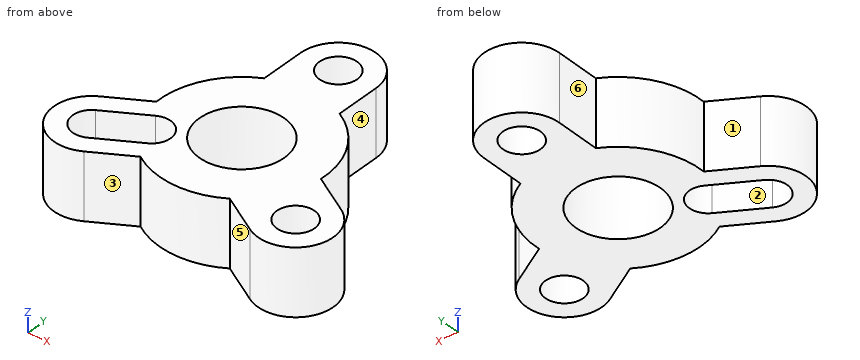
from build123d import *

# Parameters (mm, degrees)
SKETCH_1_R      = 9
SKETCH_1_R_2    = 4
EXTRUDE_1_DEPTH = 14


with BuildPart() as part:
    # Эскиз1 → Бобышка-Вытянуть1 (new body)
    with BuildSketch(Plane.XY):
        with BuildLine():
            Line((-8, 25), (-8, 15.564382416))
            ThreePointArc((-8, 15.564382416), (-15.155444566, 8.75), (-17.479150567, -0.853987978))
            Line((-17.479150567, -0.853987978), (-25.650635095, -5.57179677))
            ThreePointArc((-25.650635095, -5.57179677), (-28.578838325, -16.5), (-17.650635095, -19.42820323))
            Line((-17.650635095, -19.42820323), (-9.479150567, -14.710394438))
            ThreePointArc((-9.479150567, -14.710394438), (0, -17.5), (9.479150567, -14.710394438))
            Line((9.479150567, -14.710394438), (17.650635095, -19.42820323))
            ThreePointArc((17.650635095, -19.42820323), (28.578838325, -16.5), (25.650635095, -5.57179677))
            Line((25.650635095, -5.57179677), (17.479150567, -0.853987978))
            ThreePointArc((17.479150567, -0.853987978), (15.155444566, 8.75), (8, 15.564382416))
            Line((8, 15.564382416), (8, 25))
            ThreePointArc((8, 25), (0, 33), (-8, 25))
        make_face()
        Circle(SKETCH_1_R, mode=Mode.SUBTRACT)
        with Locations((0, 25)):
            Circle(SKETCH_1_R_2, mode=Mode.SUBTRACT)
        with Locations((21.650635095, -12.5)):
            Circle(SKETCH_1_R_2, mode=Mode.SUBTRACT)
        with BuildLine():
            Line((-14.990381057, -4.035898385), (-23.650635095, -9.035898385))
            ThreePointArc((-23.650635095, -9.035898385), (-25.11473671, -14.5), (-19.650635095, -15.964101615))
            Line((-19.650635095, -15.964101615), (-10.990381057, -10.964101615))
            ThreePointArc((-10.990381057, -10.964101615), (-9.526279442, -5.5), (-14.990381057, -4.035898385))
        make_face(mode=Mode.SUBTRACT)
    extrude(amount=EXTRUDE_1_DEPTH)


solid = part.part
Can you work these out from the model? Positions are in its coordinate system, mm. Face numbers are marked on the shaded views. A direction names the side the tool comes from. Round coordinates to 2 decimals unless told otherwise and drop trailing zeros. Write each loop counter-clockwise with the first axis right and the second up, starting at its lowest first coordinate (ties: lowest second). Pieces come first, ordered by that corner, then holes. Notation, with made-up numbers: M 26,-8 L 71,-8 A20 ccw 71,21 Z; hole C -21.5,55.25 d3. An arc over 180 degrees is marked long. Use CSV: the item, a comma, the result in double quotes.
(1) We'd pull the mould along X, two halves only. Please class the marked faces 4, 5 and 6: +X half, -X half, draft (parallel to the pull), parting line (faces both ways), or undercut.
Check values:
face 4,"+X half"
face 5,"undercut"
face 6,"-X half"
(2) Imagine slicing it at A-A (z = 1.5). Write out the boundary of the cut face in (x, y).
Check values:
outline,"M -25.65,-5.57 A8 ccw -17.65,-19.43 L -9.48,-14.71 A17.5 ccw 9.48,-14.71 L 17.65,-19.43 A8 ccw 25.65,-5.57 L 17.48,-0.85 A17.5 ccw 8,15.56 L 8,25 A8 ccw -8,25 L -8,15.56 A17.5 ccw -17.48,-0.85 Z; hole M -23.65,-9.04 A4 ccw -19.65,-15.96 L -10.99,-10.96 A4 ccw -14.99,-4.04 Z; hole C 0,0 d18; hole C 0,25 d8; hole C 21.65,-12.5 d8"
(3) I'm going to push flat-ended pins straight in: pin 1 (1 mm diameter, centred on x = -15, z = 4.5, fed in from -Y); pin 2 (4 mm diameter, centred on y = -8.5, z = 3, fed in from -X); pin 3 (2 mm diameter, centred on x = 15, z = 12.5, fed in from -Y). Where does each tip first touch, or does it pass through?
Check values:
pin 1,"y = -18.19"
pin 2,"x = -29.4"
pin 3,"y = -18.48"
(4) On a 3-axis mill with a long thin cutter (end or side, diameter ignored), from which of +Z, -Z, +X, -X, +Y, -Y can I reach the whole of each face in a straight line? I mean the marked faces 1, 2 and 3. Say none if no direction works.
Check values:
face 1,"+Z, -Z, -X, +Y"
face 2,"+Z, -Z"
face 3,"+Z, -Z, -Y"
(5) Imagine slicing it at D-D (x = 23.5). Write out the boundary of the cut face in (y, z), plus the area to 3 significant figures.
Check values:
outline,"M -20.28,0 L -16.05,0 L -16.05,14 L -20.28,14 Z; M -8.95,0 L -4.33,0 L -4.33,14 L -8.95,14 Z"
area,"124 mm^2"
(6) Imagine slicing it at C-C (y = 0). Write out the boundary of the cut face in (x, z), plus the area to 3 significant figures.
Check values:
outline,"M -17.5,0 L -9,0 L -9,14 L -17.5,14 Z; M 9,0 L 17.5,0 L 17.5,14 L 9,14 Z"
area,"238 mm^2"
(7) I need wall thicknesses on line 1 along Y through (x, z) = (0, 3.5); line 2 along X through (y, z) = (-13.5, 12.25); line 3 along X through (y, z) = (-0.5, 6.5). Which ranges of each line are inside material? Lowest first, please.
Check values:
line 1,"-17.5 to -9, 9 to 21, 29 to 33"
line 2,"-29.59 to -25.52, -15.38 to 17.78, 25.52 to 29.59"
line 3,"-17.49 to -8.99, 8.99 to 17.49"
(8) Imagine slicing it at B-B (x = 0). Write out the boundary of the cut face in (y, z).
Check values:
outline,"M -17.5,0 L -9,0 L -9,14 L -17.5,14 Z; M 9,0 L 21,0 L 21,14 L 9,14 Z; M 29,0 L 33,0 L 33,14 L 29,14 Z"
